Source: CAD feature listing. Evaluate the final solid. Frame: model axes, mm. A direction names the side the tool comes from. Give positions to 0.01 mm unless a question says otherwise; leave off trailing zeros. Order: outer loops, then holes, each group sorted by start corner. A loop starts at its lowest first (then second) coordinate and runs counter-clockwise, first axis right, second up. Notation, with made-up numbers: (88.25, 82.25) -> (123.25, 82.25) arc R28 ccw to (123.25, 114.25) -> close; hole circle Ø11 at (-20, 45.25). An arc over 180 degrees is marked (long way). Answer in a Markdown table with one row per item.
Autodesk Inventor part; units mm, degrees
ref_plane "YZ Plane" through (0, 0, 0) normal (1, 0, 0) x (0, 1, 0)
ref_plane "XZ Plane" through (0, 0, 0) normal (0, 1, 0) x (-1, 0, 0)
ref_plane "XY Plane" through (0, 0, 0) normal (0, 0, 1) x (1, 0, 0)
ref_plane "Work Plane1" through (-8.7385, 23834.0351, -280.5199) normal (0, 1, 0) x (-0.9985, 0, -0.0542)
sketch "Sketch1" plane through (-8.7385, 23834.0351, -280.5199) normal (0, 1, 0) x (-0.9985, 0, -0.0542)
  circle A0 centre (-0.1598, -60.199) radius 25.4
  circle A1 centre (-0.1598, 150.601) radius 25.4
  circle A2 centre (-0.1598, 150.601) radius 26.4
  circle A3 centre (-0.1598, -60.199) radius 26.4
  line L0 (-17.3085, -5.3414) -> (16.6915, -5.3414)
  line L1 (16.6915, -5.3414) -> (16.6915, 52.8634)
  line L2 (16.6915, 52.8634) -> (-17.3085, 52.8634)
  line L3 (-17.3085, 52.8634) -> (-17.3085, -5.3414)
  line L4 (-17.3085, 52.8634) -> (-17.3085, 130.529)
  line L5 (-17.3085, -5.3414) -> (-17.3085, -40.1271)
  line L6 (16.6915, -5.3414) -> (16.6915, -39.8768)
  line L7 (16.6915, 52.8634) -> (16.6915, 130.2787)
  line L8 (31.4252, -66.238) -> (7.3835, -90.2796)
  line L9 (7.3835, -90.2796) -> (61.8308, -144.7269)
  line L10 (61.8308, -144.7269) -> (85.8724, -120.6852)
  line L11 (85.8724, -120.6852) -> (31.4252, -66.238)
  line L12 (30.0109, -67.6522) -> (84.4582, -122.0994)
  line L13 (8.7977, -88.8654) -> (63.245, -143.3126)
  line L14 (-6.1639, -91.881) -> (-30.2055, -67.8394)
  line L15 (-30.2055, -67.8394) -> (-84.6528, -122.2866)
  line L16 (-84.6528, -122.2866) -> (-60.6111, -146.3283)
  line L17 (-60.6111, -146.3283) -> (-6.1639, -91.881)
  line L18 (-7.5781, -90.4668) -> (-62.0253, -144.914)
  line L19 (-28.7913, -69.2536) -> (-83.2386, -123.7008)
  line L20 (84.9349, 211.9974) -> (60.8933, 236.039)
  line L21 (60.8933, 236.039) -> (6.446, 181.5918)
  line L22 (6.446, 181.5918) -> (30.4877, 157.5502)
  line L23 (30.4877, 157.5502) -> (84.9349, 211.9974)
  line L24 (83.5207, 213.4116) -> (29.0735, 158.9644)
  line L25 (62.3075, 234.6248) -> (7.8603, 180.1776)
  line L26 (-32.1213, 155.9317) -> (-8.0796, 179.9733)
  line L27 (-86.5685, 210.3789) -> (-32.1213, 155.9317)
  line L28 (-85.1543, 211.7931) -> (-30.707, 157.3459)
  line L29 (-62.5268, 234.4205) -> (-86.5685, 210.3789)
  line L30 (-63.9411, 233.0063) -> (-9.4938, 178.5591)
  line L31 (-8.0796, 179.9733) -> (-62.5268, 234.4205)
  line L32 (-7.5781, -90.4668) -> (-3.4984, -86.3871)
  line L33 (-6.1639, -91.881) -> (-0.8723, -86.5894)
  line L34 (-30.2055, -67.8394) -> (-26.295, -63.9289)
  line L35 (-28.7913, -69.2536) -> (-25.8437, -66.306)
  line L36 (31.4252, -66.238) -> (26.2268, -61.0397)
  line L37 (30.0109, -67.6522) -> (26.0131, -63.6544)
  line L38 (8.7977, -88.8654) -> (5.8404, -85.9081)
  line L39 (7.3835, -90.2796) -> (3.1788, -86.3871)
  line L40 (29.0735, 158.9644) -> (25.7539, 155.6448)
  line L41 (30.4877, 157.5502) -> (26.1142, 153.1768)
  line L42 (7.8603, 180.1776) -> (4.3036, 176.6209)
  line L43 (6.446, 181.5918) -> (1.7836, 176.9293)
  line L44 (-8.0796, 179.9733) -> (-4.7119, 176.6056)
  line L45 (-9.4938, 178.5591) -> (-7.0269, 176.0922)
  line L46 (-30.707, 157.3459) -> (-26.443, 153.0818)
  line L47 (-32.1213, 155.9317) -> (-26.5588, 150.3692)
  point P0 (-23.9414, 279.6329)
  point P1 (-30.2055, -67.8394)
  dimension "d3" = 52.8
  dimension "d4" = 52.8
  dimension "d0" = 50.8
  dimension "d1" = 50.8
  dimension "d2" = 210.8
  dimension "d9" = 34
  dimension "d18" = 34
  dimension "d19" = 77
  dimension "d20" = 2
  dimension "d21" = 2
  dimension "d22" = 34
  dimension "d23" = 77
  dimension "d24" = 2
  dimension "d25" = 2
  dimension "d26" = 34
  dimension "d27" = 77
  dimension "d28" = 2
  dimension "d29" = 2
  dimension "d30" = 34
  dimension "d31" = 77
  dimension "d32" = 2
  dimension "d33" = 2
extrude "Extrusion1" add sketch "Sketch1" along normal blind 2 contours A0 | A1
extrude "Extrusion2" add sketch "Sketch1" along normal blind 23 contours A2 L26 | A3 | A2 L26
extrude "Extrusion3" add sketch "Sketch1" along normal blind 23 contours L7 L2 L4 A2 | L1 L0 L3 L2 | L6 A3 L5 L0
extrude "Extrusion4" add sketch "Sketch1" along normal blind 23 contours A2 L40 L22 L41 | L22 L24 L20 L23 | A2 L43 L22 L42 | L47 L26 L46 A2 | L22 L21 L20 L25 | L27 L29 L28 L26 | A2 L45 L26 L44 | L26 L30 L29 L31 | A3 L35 L14 L34 | L36 L8 L37 A3 | L14 L19 L16 L15 | L11 L10 L12 L8 | A3 L33 L14 L32 | L38 L8 L39 A3 | L14 L17 L16 L18 | L13 L10 L9 L8
sketch "Sketch2" plane through (-8.7385, 23857.0351, -280.5199) normal (0, 1, 0) x (0.9985, 0, 0.0542)
  line L0 (-83.5207, -213.4116) -> (-25.7539, -155.6448)
  arc A0 (-25.7539, -155.6448) -> (-4.3036, -176.6209) centre (0.1598, -150.601) ccw
  line L1 (-4.3036, -176.6209) -> (-62.3075, -234.6248)
  line L2 (63.9411, -233.0063) -> (7.0269, -176.0922)
  arc A1 (7.0269, -176.0922) -> (26.443, -153.0818) centre (0.1598, -150.601) ccw
  line L3 (26.443, -153.0818) -> (85.1543, -211.7931)
  line L4 (-26.0131, 63.6544) -> (-84.4582, 122.0994)
  arc A2 (-5.8404, 85.9081) -> (-26.0131, 63.6544) centre (0.1598, 60.199) ccw
  line L5 (-63.245, 143.3126) -> (-5.8404, 85.9081)
  line L6 (3.4984, 86.3871) -> (62.0253, 144.914)
  arc A3 (25.8437, 66.306) -> (3.4984, 86.3871) centre (0.1598, 60.199) ccw
  line L7 (83.2386, 123.7008) -> (25.8437, 66.306)
  line L8 (62.0253, 144.914) -> (83.2386, 123.7008)
  line L9 (-84.4582, 122.0994) -> (-85.8724, 120.6852)
  line L10 (-63.245, 143.3126) -> (-84.4582, 122.0994)
  line L11 (-4.3036, -176.6209) -> (-62.3075, -234.6248)
  line L12 (-62.3075, -234.6248) -> (-83.5207, -213.4116)
  line L13 (-83.5207, -213.4116) -> (-25.7539, -155.6448)
  line L14 (63.9411, -233.0063) -> (85.1543, -211.7931)
  point P0 (23.9414, -279.6329)
  point P1 (62.0253, 144.914)
  point P2 (-83.5207, -213.4116)
extrude "Extrusion5" add sketch "Sketch2" against normal blind 2
properties part number "Base"
(1) Section query A-A (z = -139.5). Return the cut outline in (x, y), plus the area to 3 significant figures.
A:
| item | result |
|---|---|
| outline | (-41.42, 23834.04) -> (7.94, 23834.04) -> (7.94, 23857.04) -> (6.87, 23857.04) -> (6.87, 23836.04) -> (-40.35, 23836.04) -> (-40.35, 23857.04) -> (-41.42, 23857.04) -> close |
| area | 144 mm^2 |
(2) Pull-direction query (X, two-part tool) for faces 5 (the flat face through (-10, 23834.035, -235)), 6 (the cylindrical face through (-24.044, 23844.388, -359.229)), 7 (the cylindrical face through (-40.652, 23845.374, -141.323)); classes: +X half, -X half, draft (parallel to the pull), parting line (faces both ways), or undercut.
A:
| item | result |
|---|---|
| face 5 | draft |
| face 6 | undercut |
| face 7 | -X half |
(3) Access query for faces 1 (the flat face through (6.16, 23845.37, -235.64)), 2 (the flat face through (-73.723, 23844.388, -98.843)), 3 (the flat face through (-27.79, 23845.37, -237.48)), 4 (the cylindrical face through (-29.216, 23846.388, -152.258)). Directions: +Z, -Z, +X, -X, +Y, -Y. A direction counts if a zero-diameter tool reaches every point of the face in a straight line with its end or side. Return the directions, or none.
A:
| item | result |
|---|---|
| face 1 | +X, +Y, -Y |
| face 2 | -Y |
| face 3 | -X, +Y, -Y |
| face 4 | +Y |
(4) Ray query, probe 1 along Z at (x, y) = (59, 23854); probe 2 along Z at (x, y) = (-18, 23850.75); probe 3 along Z at (x, y) = (-8, 23849). Return the intervals inside material, ascending.
A:
| item | result |
|---|---|
| probe 1 | z = -422.71 to -420.02, -379.72 to -377.03, -73.9 to -70.9 |
| probe 2 | z = -378.63 to -375.63, -363.78 to -362.63, -318.62 to -155.5, -104.76 to -103.76 |
| probe 3 | z = -367.75 to -365.88, -315.36 to -153.98, -106.28 to -105.22, -100.66 to -97.67 |
(5) First-contact query: pin 1 Ø8 at (x, y) = (-40, 23851.5) entering from +Z; pin 2 Ø15 at (x, z) = (1, -337) entering from +Y; pin 3 Ø8 at (x, y) = (-85.5, 23848.5) entering from -Z. Flat tips, straight axial feed; report the tip coordinate or a pass-through.
A:
| item | result |
|---|---|
| pin 1 | stops at z = -82.52 |
| pin 2 | stops at y = 23836.04 |
| pin 3 | stops at z = -407.02 |
(6) Section query B-B (z = -337). Return the cut outline in (x, y).
A:
| item | result |
|---|---|
| outline | (-31.47, 23834.04) -> (20.83, 23834.04) -> (20.83, 23857.04) -> (19.82, 23857.04) -> (19.82, 23836.04) -> (-30.46, 23836.04) -> (-30.46, 23857.04) -> (-31.47, 23857.04) -> close |
